Design review of the part built by this model. Coordinates are the model's own, in mm. Face numbers are marked on the shaded views. A direction names the side the tool comes from. Coordinates: 2 decimals unless noted, no trailing zeros. Loops run counter-clockwise (first coordinate to the right, second up) from the corner with the lowest first, then second, coordinate; pieces in that order, holes last.
Q1. Add section A-A on x = 0. Give the boundary of the cut face in (y, z), and give its area (3 significant figures).
Q2. Draft analysis for pull direction X (two halves, no side actions). For the marked faces 1, 2, 3 and 4, state which applies: released by +X, released by -X, zero draft, split by the parting line, or undercut.
Q3. Add section B-B on z = 2.1. Give the boundary of the cut face in (x, y) (3 decimals), and give its area (3 significant figures).
Q4. Add section C-C on y = -6. Give the boundary of the cut face in (x, z), and give its area (3 significant figures).
Q5. For P1, Ø2.5, axis at y = -14, z = 1.5, coming from the -X side; P2, Ø5, axis at x = -1.5, y = -25.5, coming from the -Z side; P3, Ø3, axis at x = -7.5, z = 1.5, coming from the +Y side; P4, Ø6, axis at x = 0, y = -6, coming from the -Z side, all flat-tipped, find the tip position at first contact; note any pin that passes through.
Q6. Add section D-D on x = -5.5. Give the boundary of the cut face in (y, z), and give its area (3 significant figures).
Q7. Wall thickness on probe 1 along Y at (x, z) = (0, 3.7); probe 2 along Y at (x, z) = (-5.5, 3.6); probe 3 along Y at (x, z) = (4.5, 3.2): over which ranges is each line inside the solid? List them lowest first.
Q8. Machinability: for the marked faces 5, 6, 7, 8 and 9, which of the approach directions +Z, -Z, +X, -X, +Y, -Y give a long, thin tool a straight path to every point of the face, cutting with its end or side? Answer none if there is none.
```python
from build123d import *

# Parameters (mm, degrees)
ESBO_O1_R                = 1.5
ESBO_O1_R_2              = 3.65
RESSALTO_EXTRUS_O1_DEPTH = 5
CORTE_EXTRUS_O1_DEPTH    = 3


with BuildPart() as part:
    # Esbo_o1 → Ressalto-extrus_o1 (new body)
    with BuildSketch(Plane.XY):
        Polygon((-5, 0), (-5, -30), (-9, -30), (-9, -38), (9, -38), (9, -30), (5, -30), (5, 0), align=None)
        with Locations((-5.5, -34)):
            Circle(ESBO_O1_R, mode=Mode.SUBTRACT)
        with Locations((0, -6)):
            Circle(ESBO_O1_R_2, mode=Mode.SUBTRACT)
        with BuildLine():
            Line((-0.7, -20.5), (-0.7, -17.5))
            ThreePointArc((-0.7, -17.5), (0, -16.8), (0.7, -17.5))
            Line((0.7, -17.5), (0.7, -20.5))
            ThreePointArc((0.7, -20.5), (0, -21.2), (-0.7, -20.5))
        make_face(mode=Mode.SUBTRACT)
        with BuildLine():
            Line((5.5, -32.5), (3.5, -32.5))
            ThreePointArc((3.5, -32.5), (2, -34), (3.5, -35.5))
            Line((3.5, -35.5), (5.5, -35.5))
            ThreePointArc((5.5, -35.5), (7, -34), (5.5, -32.5))
        make_face(mode=Mode.SUBTRACT)
    extrude(amount=RESSALTO_EXTRUS_O1_DEPTH)

    # Esbo_o1_3 → Corte-extrus_o1 (cut)
    with BuildSketch(Plane.XY):
        with BuildLine():
            ThreePointArc((-2.238721733, -20.225), (0, -22.25), (2.238721733, -20.225))
            Line((2.238721733, -20.225), (3.631704145, -6.365))
            ThreePointArc((3.631704145, -6.365), (0, -9.65), (-3.631704145, -6.365))
            Line((-3.631704145, -6.365), (-2.238721733, -20.225))
        make_face()
        with BuildLine():
            ThreePointArc((0.7, -20.5), (0, -21.2), (-0.7, -20.5))
            Line((-0.7, -20.5), (-0.7, -17.5))
            ThreePointArc((-0.7, -17.5), (0, -16.8), (0.7, -17.5))
            Line((0.7, -17.5), (0.7, -20.5))
        make_face(mode=Mode.SUBTRACT)
    extrude(amount=CORTE_EXTRUS_O1_DEPTH, mode=Mode.SUBTRACT)


solid = part.part
```
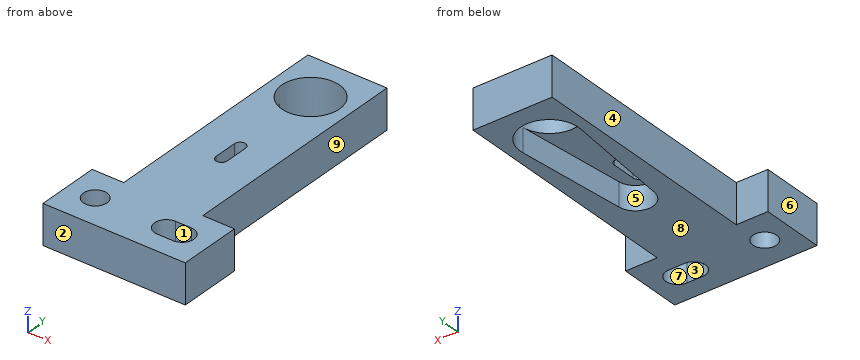
Entries:
1. outline: (-38, 0) - (-22.25, 0) - (-22.25, 3) - (-21.2, 3) - (-21.2, 5) - (-38, 5) - close; (-16.8, 3) - (-9.65, 3) - (-9.65, 5) - (-16.8, 5) - close; (-2.35, 0) - (0, 0) - (0, 5) - (-2.35, 5) - close
1. area: 107 mm2
2. face 1: undercut
2. face 2: zero draft
2. face 3: undercut
2. face 4: released by -X
3. outline: (-9, -38) - (9, -38) - (9, -30) - (5, -30) - (5, 0) - (-5, 0) - (-5, -30) - (-9, -30) - close; hole circle Ø3 at (-5.5, -34); hole (-3.632, -6.365) - (-2.239, -20.225) arc R2.25 ccw to (2.239, -20.225) - (3.632, -6.365) arc R3.65 ccw (long way) to start; hole (3.5, -35.5) - (5.5, -35.5) arc R1.5 ccw to (5.5, -32.5) - (3.5, -32.5) arc R1.5 ccw to start
3. area: 312 mm2
4. outline: (-5, 0) - (-3.65, 0) - (-3.65, 5) - (-5, 5) - close; (3.65, 0) - (5, 0) - (5, 5) - (3.65, 5) - close
4. area: 13.5 mm2
5. P1: stops at x = -5
5. P2: stops at z = 0
5. P3: stops at y = -30
5. P4: passes through
6. outline: (-38, 0) - (-35.5, 0) - (-35.5, 5) - (-38, 5) - close; (-32.5, 0) - (-30, 0) - (-30, 5) - (-32.5, 5) - close
6. area: 25.0 mm2
7. probe 1: y = -38 to -21.2, -16.8 to -9.65, -2.35 to 0
7. probe 2: y = -38 to -35.5, -32.5 to -30
7. probe 3: y = -38 to -35.5, -32.5 to 0
8. face 5: -Z
8. face 6: +Z, -Z, -X, +Y, -Y
8. face 7: +Z, -Z
8. face 8: -Z, +X, -X, +Y, -Y
8. face 9: +Z, -Z, +X, +Y
